Autodesk Inventor part; units mm, degrees
ref_plane "YZ Plane" through (0, 0, 0) normal (1, 0, 0) x (0, 1, 0)
ref_plane "XZ Plane" through (0, 0, 0) normal (0, 1, 0) x (-1, 0, 0)
ref_plane "XY Plane" through (0, 0, 0) normal (0, 0, 1) x (1, 0, 0)
sketch "Sketch1" plane through (0, 0, 0) normal (1, 0, 0) x (0, 1, 0)
  circle A0 centre (0, 0) radius 12.7
  dimension "d0" = 25.4
extrude "Extrusion1" add sketch "Sketch1" along normal blind 254
sketch "Sketch2" plane through (0, 0, 0) normal (0, 0, 1) x (1, 0, 0)
  circle A0 centre (12.7, 0) radius 6.35
  line L0 (0, 12.7) -> (0, -12.7)
  dimension "d3" = 12.7
  dimension "d4" = 12.7
extrude "Extrusion2" cut sketch "Sketch2" along normal mid plane 25.4
sketch "Sketch3" plane through (254, 0, 0) normal (1, 0, 0) x (0, 0, -1)
  circle A0 centre (0, 0) radius 6.35
  dimension "d7" = 12.7
extrude "Extrusion3" cut sketch "Sketch3" against normal blind 228.6
properties material "Aluminum 6061"
Can you work these out from the model? Positions are in its coordinate system, mm. A direction names the side the tool comes from. Coordinates: 2 decimals unless noted, no trailing zeros. Order: outer loops, then holes, each group sorted by start corner. A loop starts at its lowest first (then second) coordinate and runs counter-clockwise, first axis right, second up. Notation, with made-up numbers: (77.25, 48.5) -> (82.25, 48.5) arc R20 ccw to (82.25, 63.5) -> close; hole circle Ø3 at (44.25, 30.25). An arc over 180 degrees is marked (long way). Use one line per item in the form item = value.
Q1. Imagine slicing it at B-B, the plane y = 0. List the corners of the cut face in (x, z) for me, then the cut area to 3 significant figures.
From the geometry:
outline = (0, -12.7) -> (6.35, -12.7) -> (6.35, 12.7) -> (0, 12.7) -> close; (19.05, -12.7) -> (254, -12.7) -> (254, -6.35) -> (25.4, -6.35) -> (25.4, 6.35) -> (254, 6.35) -> (254, 12.7) -> (19.05, 12.7) -> close
area = 3,230 mm²
Q2. Imagine slicing it at C-C, the plane x = 166. List the corners of the cut face in (y, z) for me.
From the geometry:
outline = circle Ø25.4 at (0, 0); hole circle Ø12.7 at (0, 0)
Q3. I need wall thicknesses on L1, parallel to X at y = 0, z = -2.25; L2, parallel to X at y = 2.5, z = -8.25; L3, parallel to Z at x = 29.5, y = 11. Which ranges of each line are inside material? Lowest first, please.
From the geometry:
L1 = 0 to 6.35, 19.05 to 25.4
L2 = 0 to 6.86, 18.54 to 254
L3 = -6.35 to 6.35
Q4. We'd pull the mould along Y, two halves only. Please class faces 3 (the face through (125.222, -1.653, -12.592)), 4 (the face through (16.114, -5.354, -0.178)), 5 (the face through (0, 0, 0)): released by +Y, released by -Y, zero draft, split by the parting line, or undercut.
From the geometry:
face_3 = split by the parting line
face_4 = undercut
face_5 = zero draft
Q5. Which directions (+Z, -Z, +X, -X, +Y, -Y) give clear straight access to the entire face, cutting with the end or side of a thin tool? Please do faces 1 (the face through (254, 3, 6)), 2 (the face through (141.3, -6.2, 1.38)).
From the geometry:
face_1 = +Z, -Z, +X, +Y, -Y
face_2 = +X
Q6. Will these pins go through, and if not, where does the flat tip stop? P1, Ø1, axis at y = -2.5, z = 3, coming from the +X side; P2, Ø3, axis at x = 141.5, z = -5, coming from the -Y side; P3, Ø8, axis at x = 51, y = 9.5, coming from the -Z side; P4, Ø8, axis at y = -6, z = 0, coming from the -X side.
From the geometry:
P1 = 25.4
P2 = -12.21
P3 = -11.45
P4 = 0
Q7. Imagine slicing it at D-D, the plane x = 12.7. List the corners of the cut face in (y, z) for me.
From the geometry:
outline = (-6.35, -11) -> (-6.35, 11) arc R12.7 ccw to start; (6.35, -11) arc R12.7 ccw to (6.35, 11) -> close
Q8. Imagine slicing it at A-A, the plane z = 0. List the corners of the cut face in (x, y) for me.
From the geometry:
outline = (0, -12.7) -> (254, -12.7) -> (254, -6.35) -> (25.4, -6.35) -> (25.4, 6.35) -> (254, 6.35) -> (254, 12.7) -> (0, 12.7) -> close; hole circle Ø12.7 at (12.7, 0)
